CAD build for the part. Positions are in the model's coordinates, mm. Give positions to 0.01 mm unless a question says otherwise; leave off trailing zeros. Order: outer loops, then holes, each group sorted by start corner. A loop starts at its lowest first (then second) coordinate and runs counter-clockwise, first axis right, second up.
```python
from build123d import *

# Parameters (mm, degrees)
BASPROSKE_W              = 12.7
BASPROSKE_H              = 12.7
TOOTHCUT_DEPTH           = 22.997045256
TEETHCUTS_COUNT          = 10
SKETCH15_R               = 7.62
BOSS_EXTRUDE2_DEPTH      = 4.318
SKETCH8_R                = 9.2075
BOSS_EXTRUDE1_DEPTH      = 10
M2_CLEARANCE_HOLE1_D     = 2.4
M2_CLEARANCE_HOLE1_DEPTH = 10
CIRPATTERN1_COUNT        = 4
SKETCH13_R               = 4
CUT_EXTRUDE1_DEPTH       = 33.232032369
CUT_EXTRUDE1_DEPTH_BACK  = 33.232032369


with BuildPart() as part:
    # BasProSke → Base-Revolve (revolve)
    with BuildSketch(Plane(origin=(0, 0, 0), x_dir=(1, 0, 0), z_dir=(0, 1, 0)), mode=Mode.PRIVATE) as base_revolve_sk:
        with Locations((6.35, 6.35)):
            Rectangle(BASPROSKE_W, BASPROSKE_H)
    revolve(base_revolve_sk.sketch.rotate(Axis((-10, 0, 0), (1, 0, 0)), 180), axis=Axis((-10, 0, 0), (1, 0, 0)))

    # TooCutSke → ToothCut (cut, through all)
    with BuildSketch(Plane(origin=(0, 0, 0), x_dir=(0, 0, -1), z_dir=(1, 0, 0))):
        with BuildLine():
            ThreePointArc((1.261053733, 7.835399804), (0, 7.93623), (-1.261053733, 7.835399804))
            ThreePointArc((-1.261053733, 7.835399804), (-1.789991322, 10.402889218), (-3.729263267, 12.166692264))
            ThreePointArc((-3.729263267, 12.166692264), (0, 12.7254), (3.729263267, 12.166692264))
            ThreePointArc((3.729263267, 12.166692264), (1.789991322, 10.402889218), (1.261053733, 7.835399804))
        make_face()
    toothcut = extrude(amount=TOOTHCUT_DEPTH, mode=Mode.SUBTRACT)

    # TeethCuts: ToothCut ×10 about axis
    teethcuts_axis = Axis((0, 0, 0), (1, 0, 0))
    for i in range(1, TEETHCUTS_COUNT):
        add(toothcut.rotate(teethcuts_axis, i * 360 / TEETHCUTS_COUNT), mode=Mode.SUBTRACT)

    # Sketch15 → Boss-Extrude2 (add)
    with BuildSketch(Plane(origin=(12.7, 0, 0), x_dir=(0, 0, -1), z_dir=(1, 0, 0))):
        with Locations(Location((0, 0, 0), (0, 0, 180))):
            Circle(SKETCH15_R)
    extrude(amount=BOSS_EXTRUDE2_DEPTH)

    # Sketch8 → Boss-Extrude1 (add)
    with BuildSketch(Plane(origin=(17.018, 0, 0), x_dir=(0, 0, -1), z_dir=(1, 0, 0))):
        Circle(SKETCH8_R)
    extrude(amount=BOSS_EXTRUDE1_DEPTH)

    # M2 Clearance Hole1
    with Locations(Plane(origin=(27.018, 0, 0), x_dir=(0, 0, -1), z_dir=(1, 0, 0))):
        with Locations((-2.085864712, 6.419631485)):
            m2_clearance_hole1 = Hole(M2_CLEARANCE_HOLE1_D / 2, depth=M2_CLEARANCE_HOLE1_DEPTH)

    # CirPattern1: M2 Clearance Hole1 ×4 about axis, 2 skipped
    cirpattern1_axis = Axis((27.018, 0, 0), (-1, 0, 0))
    add([m2_clearance_hole1.rotate(cirpattern1_axis, i * 360 / CIRPATTERN1_COUNT) for i in range(1, CIRPATTERN1_COUNT) if i not in (1, 3)], mode=Mode.SUBTRACT)

    # Sketch13 → Cut-Extrude1 (cut, two sides)
    with BuildSketch(Plane.ZY) as cut_extrude1_sk:
        Circle(SKETCH13_R)
    extrude(amount=CUT_EXTRUDE1_DEPTH, mode=Mode.SUBTRACT)
    extrude(cut_extrude1_sk.sketch, amount=-CUT_EXTRUDE1_DEPTH_BACK, mode=Mode.SUBTRACT)


solid = part.part
```
Item 1: Two-plate mould, pull along Z, no slides. Class faces 1 (the face through (6.26, -10.42, 1.8)), 2 (the face through (0, -3, 3)), 3 (the face through (14.829, -7.555, -0.992)): released by +Z, released by -Z, zero draft, split by the parting line, or undercut.
Item 2: Slice it at B-B (y = -10). Give the cut face in (x, z), and give its area (3 significant figures).
Item 3: Slice it at D-D (x = 13.5). Give the cut face in (y, z).
Item 4: Slice it at C-C (y = 8.5). Give the cut face in (x, z), and give its area (3 significant figures).
Item 5: Slice it at A-A (z = 0). Give the cut face in (x, y), and give its area (3 significant figures).
Item 6: Drop flat-ended pins along their axis: pin 1 Ø10.5 at (y, z) = (0, 0) entering from -X; pin 2 Ø8 at (x, z) = (5.5, -8) entering from +Y; pin 3 Ø0.7 at (y, z) = (-6, -2.5) entering from +X; pin 4 Ø1 at (x, z) = (19.5, 9) entering from +Y. Give the stop position or say it passes through.
Item 7: Wall check: L1, parallel to Y at x = 21.25, z = -2; L2, parallel to Z at x = 11.75, y = 6.25; L3, parallel to Y at x = 3.25, z = 8.25. Give the ranges that are in metal, low to high.
A:
1. face 1: undercut
1. face 2: zero draft
1. face 3: split by the parting line
2. outline: (0, -4.69) - (12.7, -4.69) - (12.7, -1.59) - (0, -1.59) - close; (0, 1.59) - (12.7, 1.59) - (12.7, 4.69) - (0, 4.69) - close
2. area: 78.8 mm2
3. outline: circle Ø15.24 at (0, 0); hole circle Ø8 at (0, 0)
4. outline: (0, -4.44) - (12.7, -4.44) - (12.7, -1.24) - (0, -1.24) - close; (0, 1.24) - (12.7, 1.24) - (12.7, 4.44) - (0, 4.44) - close; (17.02, -3.54) - (27.02, -3.54) - (27.02, 3.54) - (17.02, 3.54) - close
4. area: 152 mm2
5. outline: (0, -7.94) - (12.7, -7.94) - (12.7, -7.62) - (17.02, -7.62) - (17.02, -9.21) - (27.02, -9.21) - (27.02, -4) - (0, -4) - close; (0, 4) - (27.02, 4) - (27.02, 9.21) - (17.02, 9.21) - (17.02, 7.62) - (12.7, 7.62) - (12.7, 7.94) - (0, 7.94) - close
5. area: 235 mm2
6. pin 1: stops at x = 0
6. pin 2: stops at y = 12.05
6. pin 3: stops at x = 17.02
6. pin 4: stops at y = 3.54
7. L1: y = -8.99 to -7.62, -5.22 to -3.46, 3.46 to 8.99
7. L2: z = -10.16 to -6.08, -4.89 to 4.89, 6.08 to 10.16
7. L3: y = -7.61 to -4.06, -1.38 to 1.38, 4.06 to 7.61
